Read the model definition and answer for the solid it produces. Units are mm, in the model's axes. A direction names the side the tool comes from. Round coordinates to 2 decimals unless told otherwise and drop trailing zeros. Order: outer loops, then holes, each group sorted by start corner. A loop starts at its lowest first (then second) coordinate and runs counter-clockwise, first axis right, second up. Notation, with made-up numbers: (-32, 52.5) - (16, 52.5) arc R25 ccw to (16, 88.5) - close; hole circle Ø4 at (-20.5, 21). An arc over 180 degrees is marked (long way). Answer as a JSON object with one key per item and string values. Group by question number.
Q1. A cutting plane is placed at B-B on x = 179.5. Determine the outline of the cut face in (y, z), and give its area (3 significant figures).
Q2. A cutting plane is placed at D-D on y = 114. Determine the outline of the cut face in (x, z), and give its area (3 significant figures).
Q3. Consider line 1 (Z direction, x = 405, y = 52.5); line 2 (Y direction, x = 79, z = -5.25); line 3 (Y direction, x = 489, z = -7.75). Determine where each line is inside the solid, lowest interval first.
Q4. A cutting plane is placed at A-A on z = -3.75. Determine the outline of the cut face in (x, y).
Q5. A cutting plane is placed at C-C on y = 44. Determine the outline of the cut face in (x, z), and give its area (3 significant figures).
Q6. Given pin 1 Ø4.5 at (x, y) = (498, 67.5) entering from +Z; pin 2 Ø5 at (x, z) = (378.5, -11.5) entering from -Y; pin 3 Ø4.5 at (y, z) = (184.5, 1) entering from -X, each flat-ended and moving along its own axis, determine where each tip first touches the part or whether it passes through.
Q7. A tool of negligible diameter and unlimited length cuts with its end or side. For faces 1 (the flat face through (499, 70, -10)), 2 (the flat face through (247, 150, 0)), 3 (the flat face through (247, 152, 4)), from which of +Z, -Z, +X, -X, +Y, -Y can it reach the whole face along a straight path? Write none if from no direction.
```python
from build123d import *

# Parameters (mm, degrees)
BOSS_EXTRUDE1_DEPTH = 4
SKETCH2_W           = 337
SKETCH2_H           = 4
BOSS_EXTRUDE2_DEPTH = 20
BOSS_EXTRUDE3_DEPTH = 20
SKETCH7_W           = 20
SKETCH7_H           = 4
BOSS_EXTRUDE6_DEPTH = 24
SKETCH8_W           = 20
SKETCH8_H           = 4
BOSS_EXTRUDE7_DEPTH = 24
FILLET1_R           = 10


with BuildPart() as part:
    # Sketch1 → Boss-Extrude1 (new body)
    with BuildSketch(Plane.XY):
        Polygon((0, 0), (0, 300), (337, 300), (487, 70), (487, 0), align=None)
    extrude(amount=BOSS_EXTRUDE1_DEPTH)

    # Sketch2 → Boss-Extrude2 (add)
    with BuildSketch(Plane(origin=(0, 0, 0), x_dir=(-1, 0, 0), z_dir=(0, 0, -1))):
        with Locations((-168.5, 298)):
            Rectangle(SKETCH2_W, SKETCH2_H)
    extrude(amount=BOSS_EXTRUDE2_DEPTH)

    # Sketch3 → Boss-Extrude3 (add)
    with BuildSketch(Plane(origin=(0, 0, 0), x_dir=(-1, 0, 0), z_dir=(0, 0, -1))):
        Polygon((-337, 300), (-337, 296), (-487, 66), (-487, 70), align=None)
    extrude(amount=BOSS_EXTRUDE3_DEPTH)

    # Sketch7 → Boss-Extrude6 (add)
    with BuildSketch(Plane(origin=(487, 0, 0), x_dir=(0, 0, -1), z_dir=(1, 0, 0))):
        with Locations((10, 68)):
            Rectangle(SKETCH7_W, SKETCH7_H)
    extrude(amount=BOSS_EXTRUDE6_DEPTH)

    # Sketch8 → Boss-Extrude7 (add)
    with BuildSketch(Plane.ZY):
        with Locations((-10, 298)):
            Rectangle(SKETCH8_W, SKETCH8_H)
    extrude(amount=BOSS_EXTRUDE7_DEPTH)

    # Fillet1
    fillet1_edges = [part.edges().sort_by_distance(p)[0] for p in [
        (511, 68, -20),
        (-24, 298, -20),
    ]]
    fillet(fillet1_edges, radius=FILLET1_R)


solid = part.part
```
Result set:
{
 "1": {"outline": "(0, 0) - (296, 0) - (296, -20) - (300, -20) - (300, 4) - (0, 4) - close", "area": "1,280 mm²"},
 "2": {"outline": "(0, 0) - (455.7, 0) - (455.7, -20) - (458.3, -20) - (458.3, 4) - (0, 4) - close", "area": "1,890 mm²"},
 "3": {"line 1": "z = 0 to 4", "line 2": "y = 296 to 300", "line 3": "y = 66 to 70"},
 "4": {"outline": "(-24, 296) - (337, 296) - (487, 66) - (511, 66) - (511, 70) - (487, 70) - (337, 300) - (-24, 300) - close"},
 "5": {"outline": "(0, 0) - (487, 0) - (487, 4) - (0, 4) - close", "area": "1,950 mm²"},
 "6": {"pin 1": "stops at z = 0", "pin 2": "stops at y = 228.53", "pin 3": "stops at x = 0"},
 "7": {"face 1": "+Z, -Z, +X, +Y", "face 2": "-Z, -X, -Y", "face 3": "+Z, +X, -X, +Y, -Y"}
}
